from build123d import *

# Parameters (mm, degrees)
SKETCH_1_R      = 3
SKETCH_1_R_2    = 2.05
EXTRUDE_1_DEPTH = 2
CHAMFER_1_SIZE  = 0.1


with BuildPart() as part:
    # 草图1 → 凸台-拉伸1 (new body)
    with BuildSketch(Plane.YZ):
        with Locations(Location((0, 0, 0), (0, 0, 270))):
            Circle(SKETCH_1_R)
        with Locations(Location((0, 0, 0), (0, 0, 270))):
            Circle(SKETCH_1_R_2, mode=Mode.SUBTRACT)
    extrude(amount=EXTRUDE_1_DEPTH)

    # 倒角1
    chamfer_1_edges = [part.edges().sort_by_distance(p)[0] for p in [
        (0, 0, 3),
        (2, 0, 3),
        (0, 0, 2.05),
        (2, 0, 2.05),
    ]]
    chamfer(chamfer_1_edges, length=CHAMFER_1_SIZE)


solid = part.part
Read the model definition and answer for the solid it produces. Units are mm, in the model's axes. Give positions to 0.01 mm unless a question says otherwise; leave off trailing zeros. Loops run counter-clockwise (first coordinate to the right, second up) from the corner with the lowest first, then second, coordinate; pieces in that order, holes last. Notation, with made-up numbers: (-11.5, 14) - (-1.5, 14) arc R8 ccw to (-1.5, 24) - close; hole circle Ø3 at (-22, 5.5). An arc over 180 degrees is marked (long way). Answer as CSV lines item,"result". Start each with the question number.
1) Find section C-C (x = 1.6). Write down the section's boundary in (y, z).
2) Determine the mould class of faces 1 (the face through (0.987, 2.033, 0.267)), 2 (the face through (0.99, 0.9, -2.86)) for opening direction Y: released by +Y, released by -Y, zero draft, split by the parting line, or undercut.
3) Find section A-A (z = 0). Write down the section's boundary in (x, y), then the cut area to 3 significant figures.
4) This flat-tipped pin is pushed along its axis until it touches: pin 1 Ø1 at (x, z) = (0, -1.5) entering from -Y. Where does it stop, or does it pass through?
5) Straight lines are drawn through the part: L1, parallel to Y at x = 0.5, z = 0; L2, parallel to Z at x = 0.7, y = 1.8; L3, parallel to Y at x = 1.6, z = 1.65. For each, find the intervals that lie inside material, in ascending order. Write a range as from..to.
Findings below:
1,outline,"circle Ø6 at (0, 0); hole circle Ø4.1 at (0, 0)"
2,face 1,"undercut"
2,face 2,"split by the parting line"
3,outline,"(0, -2.9) - (0.1, -3) - (1.9, -3) - (2, -2.9) - (2, -2.15) - (1.9, -2.05) - (0.1, -2.05) - (0, -2.15) - close; (0, 2.15) - (0.1, 2.05) - (1.9, 2.05) - (2, 2.15) - (2, 2.9) - (1.9, 3) - (0.1, 3) - (0, 2.9) - close"
3,area,"3.76 mm^2"
4,pin 1,"y = -2.82"
5,L1,"-3..-2.05, 2.05..3"
5,L2,"-2.4..-0.98, 0.98..2.4"
5,L3,"-2.51..-1.22, 1.22..2.51"
